Input: part model. Units: mm. Frame: model coordinates. Face numbers are marked on the shaded views. Round coordinates to 2 decimals unless told otherwise and drop trailing zeros. Loops run counter-clockwise (first coordinate to the right, second up) from the corner with the lowest first, then second, coordinate; pieces in that order, holes last. Notation, with made-up numbers: (20, 49) -> (33, 49) arc R22 cw to (33, 64) -> close; hole circle Ø7 at (-14.5, -15). An arc over 180 degrees is marked (long way). Answer as a JSON object with one key per item and string values. Group by question number.
Item 1: Section query C-C on z = 2.2. Return loops of the section in (x, y).
Item 2: Material intervals for line 1 (Y direction, x = 3.75, z = 1.5); line 2 (Y direction, x = 3, z = 0.9); line 3 (Y direction, x = 0.5, z = 1.1), sorted ascending. Write a range as [from, to].
Item 3: Section query A-A on y = -24. Return loops of the section in (x, z), and give its area (3 significant figures).
Item 4: Section query B-B on x = 0.5. Return loops of the section in (y, z), and give its area (3 significant figures).
Item 5: Draft query along X for the marked faces 1, 2 and 3. Return one class per face: released by +X, released by -X, zero draft, split by the parting line, or undercut.
Item 6: Pin query (flat end, axial travel): pin 1 (4 mm diameter, centred on x = 5.5, y = 1.5, fed in from -Z). Return the tip coordinate at first contact, or that it passes through.
from build123d import *

# Parameters (mm, degrees)
CROQUIS1_W              = 24
CROQUIS1_H              = 47.5
CROQUIS1_R              = 2
CROQUIS1_R_2            = 4.25
SALIENTE_EXTRUIR1_DEPTH = 5
CORTAR_EXTRUIR2_DEPTH   = 5


with BuildPart() as part:
    # Croquis1 → Saliente-Extruir1 (new body)
    with BuildSketch(Plane.XY):
        with Locations((0, -16.25)):
            Rectangle(CROQUIS1_W, CROQUIS1_H)
        with Locations((4.5, -8)):
            Circle(CROQUIS1_R, mode=Mode.SUBTRACT)
        with Locations((4.5, -16)):
            Circle(CROQUIS1_R, mode=Mode.SUBTRACT)
        with Locations((4.5, -24)):
            Circle(CROQUIS1_R, mode=Mode.SUBTRACT)
        with Locations((0.5, 0)):
            Circle(CROQUIS1_R_2, mode=Mode.SUBTRACT)
        with Locations((4.5, -32)):
            Circle(CROQUIS1_R, mode=Mode.SUBTRACT)
    extrude(amount=SALIENTE_EXTRUIR1_DEPTH)

    # Croquis2 → Cortar-Extruir2 (cut)
    with BuildSketch(Plane(origin=(0, 0, 0), x_dir=(-1, 0, 0), z_dir=(0, 0, -1))):
        Polygon((5.5, 7.5), (12, 7.5), (12, -43.69397747), (5.5, -43.69397747), (5.5, -29.215049773), align=None)
    extrude(amount=-CORTAR_EXTRUIR2_DEPTH, mode=Mode.SUBTRACT)


solid = part.part
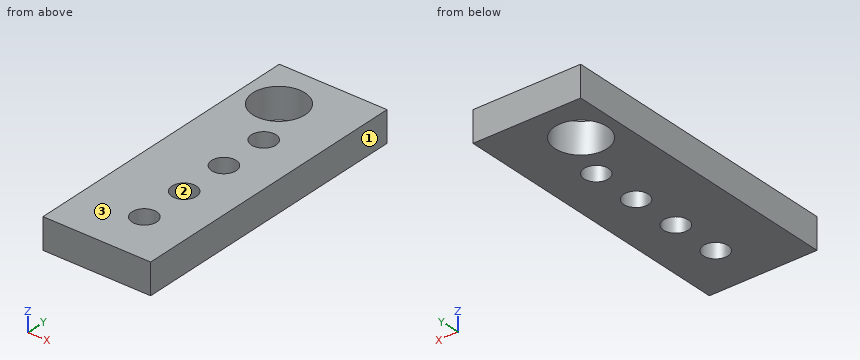
Solved:
{
 "1": {"outline": "(-5.5, -40) -> (12, -40) -> (12, 7.5) -> (-5.5, 7.5) -> close; hole circle Ø8.5 at (0.5, 0); hole circle Ø4 at (4.5, -32); hole circle Ø4 at (4.5, -24); hole circle Ø4 at (4.5, -16); hole circle Ø4 at (4.5, -8)"},
 "2": {"line 1": "[-40, -33.85], [-30.15, -25.85], [-22.15, -17.85], [-14.15, -9.85], [-6.15, -2.74], [2.74, 7.5]", "line 2": "[-40, -33.32], [-30.68, -25.32], [-22.68, -17.32], [-14.68, -9.32], [-6.68, -3.44], [3.44, 7.5]", "line 3": "[-40, -4.25], [4.25, 7.5]"},
 "3": {"outline": "(-5.5, 0) -> (2.5, 0) -> (2.5, 5) -> (-5.5, 5) -> close; (6.5, 0) -> (12, 0) -> (12, 5) -> (6.5, 5) -> close", "area": "67.5 mm²"},
 "4": {"outline": "(-40, 0) -> (-4.25, 0) -> (-4.25, 5) -> (-40, 5) -> close; (4.25, 0) -> (7.5, 0) -> (7.5, 5) -> (4.25, 5) -> close", "area": "195 mm²"},
 "5": {"face 1": "released by +X", "face 2": "undercut", "face 3": "zero draft"},
 "6": {"pin 1": "z = 0"}
}
